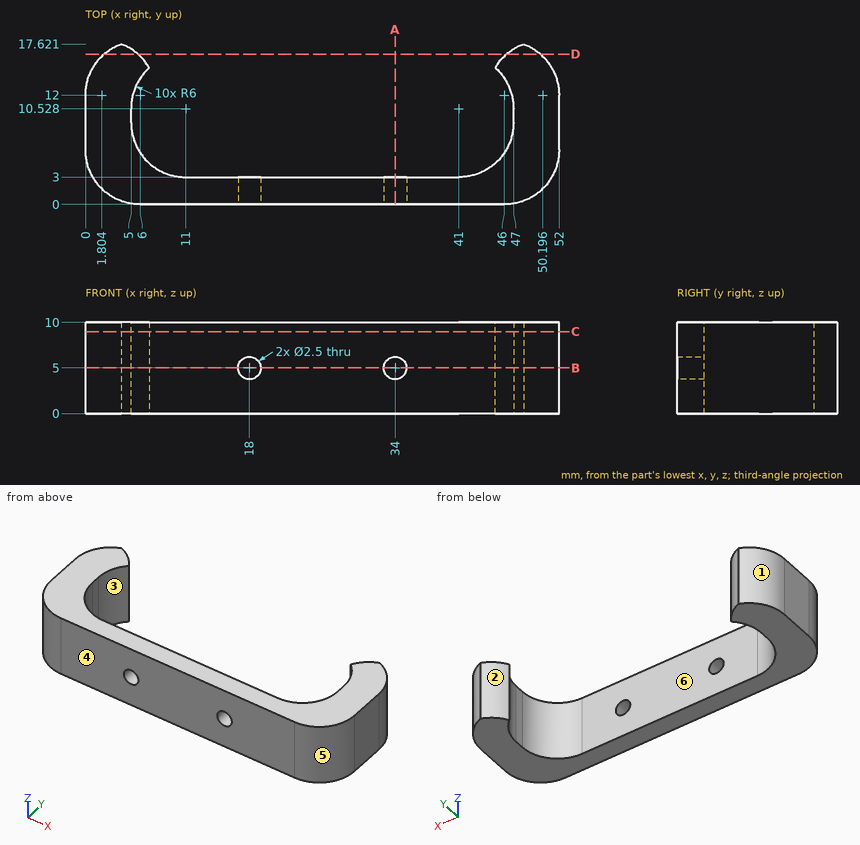
Design review of the part shown in the three views and the two pictorial views. Dimensions are in mm from the part's minimum x, y and z. A direction names the side the tool comes from. Give positions to 0.01 mm unless a question says otherwise; leave off trailing zeros. Loops run counter-clockwise (first coordinate to the right, second up) from the corner with the lowest first, then second, coordinate; pieces in that order, holes last. Notation, with made-up numbers: M 88.25,39.25 L 144.25,39.25 A31 ccw 144.25,75.25 Z; hole C 60,50 d11. An arc over 180 degrees is marked long. Answer as a JSON object with one key per item and string values. Group by question number.
Q1. Add section D-D on y = 16.5. Give the boundary of the cut face in (x, z).
Q2. Add section B-B on z = 5. Give the boundary of the cut face in (x, y).
Q3. Mouldability with a two-part tool opening along X and no side actions: class the marked faces 4, 5 and 6 as +X half, -X half, draft (parallel to the pull), parting line (faces both ways), or undercut.
Q4. Add section A-A on x = 34. Give the boundary of the cut face in (y, z), and give its area (3 significant figures).
Q5. Add section C-C on z = 9. Give the boundary of the cut face in (x, y).
Q6. Insertion check: P1, Ø3, axis at x = 18, z = 5, coming from the -Y side; P2, Ø1.5, axis at y = 14, z = 6.5, coming from the -X side; P3, Ø3, axis at x = 21, z = 6.5, coming from the +Y side; P4, Ø1.5, axis at y = 3, z = 6, coming from the -X side. Each pin has a flat end and moves straight along its axis. Give the tip position at first contact, or say it passes through.
Q7. Tool access review of the marked faces 1, 2 and 3: name each direction out of +Z, -Z, +X, -X, +Y, -Y from which nothing blocks a thin tool from reaching the whole face with its end or side.
Q8. For probe 1 along X at (y, z) = (2.35, 5); probe 2 along Z at (x, y) = (34, 0.85); probe 3 along X at (y, z) = (1.45, 5), list the stretches that pass through material, from the lowest coordinate up. Write a range as [from, to].
Checked values:
{
 "1": {"outline": "M 2.03,0 L 5.77,0 L 5.77,10 L 2.03,10 Z; M 46.23,0 L 49.97,0 L 49.97,10 L 46.23,10 Z"},
 "2": {"outline": "M 0,6 A6 ccw 6,0 L 16.75,0 L 16.75,3 L 11,3 A6 cw 5,9 L 5,10.53 A6 cw 7,15 A6 ccw 3.9,17.62 A6 ccw 0,12 Z; M 19.25,0 L 32.75,0 L 32.75,3 L 19.25,3 Z; M 35.25,0 L 46,0 A6 ccw 52,6 L 52,12 A6 ccw 48.1,17.62 A6 ccw 45,15 A6 cw 47,10.53 L 47,9 A6 cw 41,3 L 35.25,3 Z"},
 "3": {"face 4": "draft", "face 5": "+X half", "face 6": "undercut"},
 "4": {"outline": "M 0,0 L 3,0 L 3,3.75 L 0,3.75 Z; M 0,6.25 L 3,6.25 L 3,10 L 0,10 Z", "area": "22.5 mm²"},
 "5": {"outline": "M 0,6 A6 ccw 6,0 L 46,0 A6 ccw 52,6 L 52,12 A6 ccw 48.1,17.62 A6 ccw 45,15 A6 cw 47,10.53 L 47,9 A6 cw 41,3 L 11,3 A6 cw 5,9 L 5,10.53 A6 cw 7,15 A6 ccw 3.9,17.62 A6 ccw 0,12 Z"},
 "6": {"P1": "y = 0", "P2": "x = 0.13", "P3": "y = 3", "P4": "x = 0.44"},
 "7": {"face 1": "+Z, -Z, -X, +Y", "face 2": "+Z, -Z, +Y", "face 3": "+Z, -Z"},
 "8": {"probe 1": "[1.24, 16.75], [19.25, 32.75], [35.25, 50.76]", "probe 2": "[0, 3.75], [6.25, 10]", "probe 3": "[2.09, 16.75], [19.25, 32.75], [35.25, 49.91]"}
}
